Check sheet for the modelled part. Datum: model origin and axes. Units: mm. A direction names the side the tool comes from. Round coordinates to 2 decimals unless told otherwise and drop trailing zeros. Write each loop counter-clockwise with the first axis right and the second up, starting at its lowest first coordinate (ties: lowest second). Pieces come first, ordered by that corner, then holes. Notation, with made-up numbers: M -16,43.5 L 39,43.5 A26 ccw 39,78.5 Z; hole C 50,79.25 d10. An arc over 180 degrees is marked long. One line per item, written item: value.
from build123d import *

# Parameters (mm, degrees)
CUT_EXTRUDE1_DEPTH = 10.16


with BuildPart() as part:
    # Sketch1 → Revolve1 (revolve)
    with BuildSketch(Plane(origin=(0, 0, 0), x_dir=(0, 0, -1), z_dir=(1, 0, 0))):
        with BuildLine():
            Line((-5.08, -11.938), (5.08, -11.938))
            Line((5.08, -11.938), (5.08, -0.254))
            ThreePointArc((5.08, -0.254), (4.064, 0.762), (5.08, 1.778))
            Line((5.08, 1.778), (5.08, 11.938))
            Line((5.08, 11.938), (-5.08, 11.938))
            Line((-5.08, 11.938), (-5.08, 1.778))
            ThreePointArc((-5.08, 1.778), (-4.064, 0.762), (-5.08, -0.254))
            Line((-5.08, -0.254), (-5.08, -11.938))
        make_face()
    revolve(axis=Axis((0, 11.938, 5.08), (0, 0, -1)))

    # Sketch2 → Cut-Extrude1 (cut)
    with BuildSketch(Plane.XY.offset(5.08)):
        Polygon((7.332348419, 11.938), (3.666174209, 18.288), (-3.666174209, 18.288), (-7.332348419, 11.938), (-3.666174209, 5.588), (3.666174209, 5.588), align=None)
    extrude(amount=-CUT_EXTRUDE1_DEPTH, mode=Mode.SUBTRACT)


solid = part.part
Q1. Draft check along Y on faces 1 (the flat face through (-6, 1, 5.08)), 2 (the flat face through (0, 18.288, 0)), 3 (the flat face through (5.474, 8.719, 0.071)), 4 (the cylindrical face through (-7.172, -10.835, -0.071)). Enter one of: pulls with the +Y half, pulls with the -Y half, needs draft (parallel to the pull), parting line crosses it, or undercut.
Completed:
face 1: needs draft
face 2: undercut
face 3: undercut
face 4: parting line crosses it
Q2. Sectioned sample at C-C on y = 27.5. Enter the section's corners in (x, z).
Completed:
outline: M -18.11,-5.08 L 18.11,-5.08 L 18.11,5.08 L -18.11,5.08 Z
Q3. Scan lines: line 1 (X direction, y = 7.5, z = -2.25); line 2 (Z direction, x = 1.5, y = 23); line 3 (X direction, y = 15, z = 0.5). Record each from-to range of solid material in increasing order. Write a range as [from, to].
Completed:
line 1: [-23.46, -4.77], [4.77, 23.46]
line 2: [-4.06, 4.06]
line 3: [-23.68, -5.56], [5.56, 23.68]
Q4. Sectioned sample at B-B on z = -0.25. Enter the section's corners in (x, y), and give its area (3 significant figures).
Completed:
outline: C 0,11.94 d47.75; hole M -7.33,11.94 L -3.67,5.59 L 3.67,5.59 L 7.33,11.94 L 3.67,18.29 L -3.67,18.29 Z
area: 1,650 mm^2
Q5. Sectioned sample at A-A on x = 0. Enter the section's corners in (y, z).
Completed:
outline: M -11.94,-5.08 L -0.25,-5.08 A1.02 cw 1.78,-5.08 L 5.59,-5.08 L 5.59,5.08 L 1.78,5.08 A1.02 cw -0.25,5.08 L -11.94,5.08 Z; M 18.29,-5.08 L 22.1,-5.08 A1.02 cw 24.13,-5.08 L 35.81,-5.08 L 35.81,5.08 L 24.13,5.08 A1.02 cw 22.1,5.08 L 18.29,5.08 Z
Q6. Sectioned sample at D-D on y = -7.5. Enter the section's corners in (x, z).
Completed:
outline: M -13.86,-5.08 L 13.86,-5.08 L 13.86,5.08 L -13.86,5.08 Z
Q7. Access from +Z, -Z, +X, -X, +Y, -Y to the whole of each face (thin tool, end or side, straight path). Record for faces 5 (the flat face through (-6, 23, -5.08)), 6 (the flat face through (0, 5.588, 0)).
Completed:
face 5: -Z, +X, -X, +Y, -Y
face 6: +Z, -Z
Q8. Depth check by flat-ended pin: P1, Ø4, axis at y = 27, z = 2, coming from the +X side; P2, Ø3.5, axis at x = 1.5, z = -1, coming from the +Y side; P3, Ø3, axis at y = 5, z = -4, coming from the -X side; P4, Ø3, axis at x = -12, z = 0, coming from the -Y side. Enter the tip coordinate at first touch or a pass-through.
Completed:
P1: x = 19.99
P2: y = 35.81
P3: x = -23.25
P4: y = -9.51
